Could you check a few things on this model? Use its own coordinates, in mm. A direction names the side the tool comes from. Give positions to 0.01 mm unless a question says otherwise; leave off trailing zeros. Order: outer loops, then holes, each group sorted by start corner. A loop starts at its lowest first (then second) coordinate and runs counter-clockwise, first axis right, second up. Notation, with made-up numbers: M 6,-35.5 L 55,-35.5 A12 cw 55,-15.5 Z; hole C 14,33 d2. An arc over 180 degrees is marked long. Use a Markdown table: item, result. Add a question column.
```python
from build123d import *

# Parameters (mm, degrees)
SZKIC1_W                          = 16
SZKIC1_H                          = 6
DODANIE_WYCI_GNI_CIE1_DEPTH       = 6
SZKIC2_W                          = 15
SZKIC2_H                          = 5
WYTNIJ_WYCI_GNI_CIE1_DEPTH        = 5.5
SZKIC3_W                          = 2
SZKIC3_H                          = 0.5
WYTNIJ_WYCI_GNI_CIE2_DEPTH        = 18.349351573
WYTNIJ_WYCI_GNI_CIE3_REACH        = 13.662
SZKIC4_W                          = 7.5
SZKIC4_H                          = 4.5
WYTNIJ_WYCI_GNI_CIE4_REACH        = 13.662
SZKIC5_W                          = 1
SZKIC5_H                          = 2
SZKIC6_W                          = 0.45
SZKIC6_H                          = 0.45
DODANIE_WYCI_GNI_CIE2_DEPTH       = 4.75
SFAZOWANIE1_SIZE                  = 0.1
SZYK_LINIOWY1_COUNT               = 6
SZYK_LINIOWY1_PITCH               = 2.2
SFAZOWANIE1_OF_SZYK_LINIOWY1_SIZE = 0.1


with BuildPart() as part:
    # Szkic1 → Dodanie-wyciągnięcie1 (new body)
    with BuildSketch(Plane.XY):
        Rectangle(SZKIC1_W, SZKIC1_H)
    extrude(amount=DODANIE_WYCI_GNI_CIE1_DEPTH)

    # Szkic2 → Wytnij-wyciągnięcie1 (cut)
    with BuildSketch(Plane.XY.offset(6)):
        Rectangle(SZKIC2_W, SZKIC2_H)
    extrude(amount=-WYTNIJ_WYCI_GNI_CIE1_DEPTH, mode=Mode.SUBTRACT)

    # Szkic3 → Wytnij-wyciągnięcie2 (cut, through all)
    with BuildSketch(Plane(origin=(8, 0, 0), x_dir=(0, 0, -1), z_dir=(1, 0, 0))):
        with Locations((-5, -2)):
            Rectangle(SZKIC3_W, SZKIC3_H)
    extrude(amount=-WYTNIJ_WYCI_GNI_CIE2_DEPTH, mode=Mode.SUBTRACT)

    # Szkic4 → Wytnij-wyciągnięcie3 (cut, up to next)
    with BuildSketch(Plane.XZ.offset(3), mode=Mode.PRIVATE) as wytnij_wyci_gni_cie3_sk1:
        with Locations((0, 3.75)):
            Rectangle(SZKIC4_W, SZKIC4_H)
    wytnij_wyci_gni_cie3_tool1 = extrude(wytnij_wyci_gni_cie3_sk1.sketch, amount=-WYTNIJ_WYCI_GNI_CIE3_REACH, mode=Mode.PRIVATE) & part.part
    add(wytnij_wyci_gni_cie3_tool1.solids().sort_by_distance((0, -3, 3.75))[0], mode=Mode.SUBTRACT)

    # Szkic5 → Wytnij-wyciągnięcie4 (cut, up to next)
    with BuildSketch(Plane.XZ.offset(3), mode=Mode.PRIVATE) as wytnij_wyci_gni_cie4_sk1:
        with Locations((-6.75, 1.5)):
            Rectangle(SZKIC5_W, SZKIC5_H)
    wytnij_wyci_gni_cie4_tool1 = extrude(wytnij_wyci_gni_cie4_sk1.sketch, amount=-WYTNIJ_WYCI_GNI_CIE4_REACH, mode=Mode.PRIVATE) & part.part
    # Szkic5 → Wytnij-wyciągnięcie4 (cut, up to next)
    with BuildSketch(Plane.XZ.offset(3), mode=Mode.PRIVATE) as wytnij_wyci_gni_cie4_sk2:
        with Locations((6.75, 1.5)):
            Rectangle(SZKIC5_W, SZKIC5_H)
    wytnij_wyci_gni_cie4_tool2 = extrude(wytnij_wyci_gni_cie4_sk2.sketch, amount=-WYTNIJ_WYCI_GNI_CIE4_REACH, mode=Mode.PRIVATE) & part.part
    add(wytnij_wyci_gni_cie4_tool1.solids().sort_by_distance((-6.75, -3, 1.5))[0], mode=Mode.SUBTRACT)
    add(wytnij_wyci_gni_cie4_tool2.solids().sort_by_distance((6.75, -3, 1.5))[0], mode=Mode.SUBTRACT)

    # Szkic6 → Dodanie-wyciągnięcie2 (add)
    with BuildSketch(Plane.XY.offset(0.5)):
        with Locations((-5.775, 0)):
            Rectangle(SZKIC6_W, SZKIC6_H)
    dodanie_wyci_gni_cie2 = extrude(amount=DODANIE_WYCI_GNI_CIE2_DEPTH)

    # Sfazowanie1
    sfazowanie1_edges = [part.edges().sort_by_distance(p)[0] for p in [
        (-5.55, 0, 5.25),
        (-5.775, 0.225, 5.25),
        (-6, 0, 5.25),
        (-5.775, -0.225, 5.25),
    ]]
    chamfer(sfazowanie1_edges, length=SFAZOWANIE1_SIZE)

    # Szyk liniowy1: Dodanie-wyciągnięcie2 ×6
    with Locations(*[(i * SZYK_LINIOWY1_PITCH, 0, 0) for i in range(1, SZYK_LINIOWY1_COUNT)]):
        add(dodanie_wyci_gni_cie2)

    # Sfazowanie1 of Szyk liniowy1
    sfazowanie1_of_szyk_liniowy1_edges = [part.edges().sort_by_distance(p)[0] for p in [
        (-3.35, 0, 5.25),
        (-3.575, 0.225, 5.25),
        (-3.8, 0, 5.25),
        (-3.575, -0.225, 5.25),
        (-1.15, 0, 5.25),
        (-1.375, 0.225, 5.25),
        (-1.6, 0, 5.25),
        (-1.375, -0.225, 5.25),
        (1.05, 0, 5.25),
        (0.825, 0.225, 5.25),
        (0.6, 0, 5.25),
        (0.825, -0.225, 5.25),
        (3.25, 0, 5.25),
        (3.025, 0.225, 5.25),
        (2.8, 0, 5.25),
        (3.025, -0.225, 5.25),
        (5.45, 0, 5.25),
        (5.225, 0.225, 5.25),
        (5, 0, 5.25),
        (5.225, -0.225, 5.25),
    ]]
    chamfer(sfazowanie1_of_szyk_liniowy1_edges, length=SFAZOWANIE1_OF_SZYK_LINIOWY1_SIZE)


solid = part.part
```
1) Suppose I cut it at B-B on z = 0.7. Count the separate pieces of the cut face and the enclosed holes in it, and give its area (3 significant figures).
2) Suppose I cut it at C-C on y = 1.8. Please give me the cut outline in (x, z), and give its area (3 significant figures).
3) We'd pull the mould along X, two halves only. Please class faces 1 (the face through (0, -2.5, 1)), 2 (the face through (8, 0, 3)), 3 (the face through (7.5, 0, 3)), 4 (the face through (0, -3, 1)): pulls with the +X half, pulls with the -X half, needs draft (parallel to the pull), parting line crosses it, or undercut.
4) Suppose I cut it at A-A on x = 2. Please give me the cut outline in (y, z).
5) Please list where these lines run through material, in increasing order: line 1 (X direction, y = 2.2, z = 4.3); line 2 (Y direction, x = 4, z = 1.9); line 3 (Y direction, x = 3, z = 5) (3 decimals). Write a range as from..to.
6) For faces 5 (the face through (0, 2.5, 3)), 6 (the face through (-8, 0, 3)), which set-ups out of +Z, -Z, +X, -X, +Y, -Y let a thin tool reach every point of the face, with its end or its side?
Values found:
| question | item | result |
|---|---|---|
| 1 | separate pieces | 8 |
| 1 | enclosed holes | 0 |
| 1 | area | 21.2 mm^2 |
| 2 | outline | M -8,0 L 8,0 L 8,6 L 7.5,6 L 7.5,0.5 L -7.5,0.5 L -7.5,6 L -8,6 Z |
| 2 | area | 13.5 mm^2 |
| 3 | face 1 | undercut |
| 3 | face 2 | pulls with the +X half |
| 3 | face 3 | undercut |
| 3 | face 4 | needs draft |
| 4 | outline | M -3,0 L 3,0 L 3,6 L 2.5,6 L 2.5,0.5 L -2.5,0.5 L -2.5,1.5 L -3,1.5 Z |
| 5 | line 1 | x = -8..-7.5, 7.5..8 |
| 5 | line 2 | y = -3..-2.5, 2.5..3 |
| 5 | line 3 | y = -0.225..0.225, 2.5..3 |
| 6 | face 5 | +Z |
| 6 | face 6 | +Z, -Z, -X, +Y, -Y |
